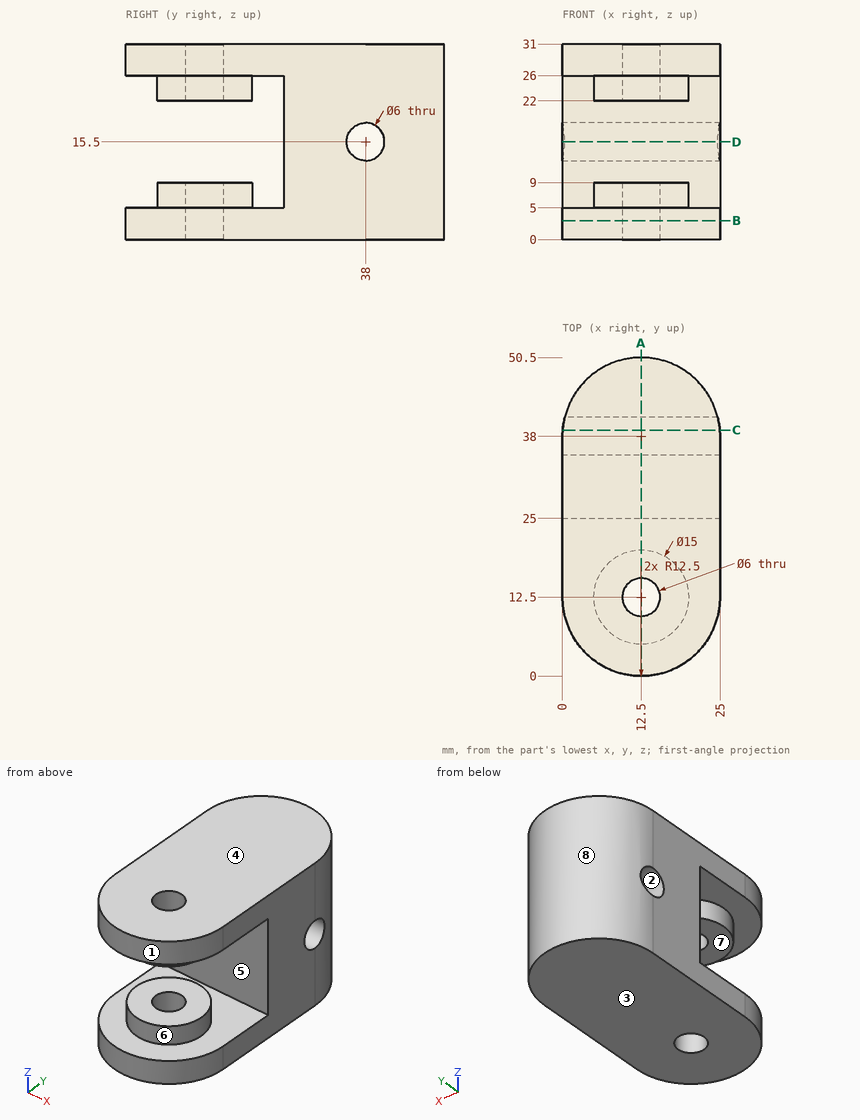
Part print with two shaded views. Sizes in mm from the minimum x, y, z corner. A direction names the side the tool comes from. Coordinates: 2 decimals unless noted, no trailing zeros. Write each loop counter-clockwise with the first axis right and the second up, starting at its lowest first coordinate (ties: lowest second). Pieces come first, ordered by that corner, then holes.
(1) Pin check, flat tips, straight feed: pin 1 Ø1 at (y, z) = (10, 26) entering from -X; pin 2 Ø5.5 at (y, z) = (38, 15.5) entering from +X; pin 3 Ø6 at (x, z) = (10, 22.5) entering from -Y. Stop position of each tip, or through.
(2) Cut at B-B on z = 3. List the corners of the cut face in (x, y), and give its area (3 significant figures).
(3) Drill centre lines: line 1 (Y direction, x = 12.5, z = 7.25); line 2 (Z direction, x = 6.25, y = 14); line 3 (Z direction, x = 20, y = 3). Where is each one in solid material? Low to high.
(4) 3-axis set-ups, long thin cutter, end or side, ignore diameter. For the marked faces 4, 5, 6, 7 and 8: which of +Z, -Z, +X, -X, +Y, -Y reach the whole face in a straight line?
(5) Mould opens along Z. For the marked faces 1, 2 and 3 say: pulls with the +Z half, pulls with the -Z half, needs draft (parallel to the pull), parting line crosses it, or undercut.
(6) Cut at D-D on z = 15.5. List the corners of the cut face in (x, y).
(7) Cut at C-C on y = 39. List the corners of the cut face in (x, z), and give its area (3 significant figures).
(8) Cut at A-A on x = 12.5. List the corners of the cut face in (y, z), and give its area (3 significant figures).
Working result:
1. pin 1: stops at x = 0.16
1. pin 2: passes through
1. pin 3: stops at y = 5
2. outline: (0, 12.5) arc R12.5 ccw to (25, 12.5) - (25, 38) arc R12.5 ccw to (0, 38) - close; hole circle Ø6 at (12.5, 12.5)
2. area: 1,100 mm2
3. line 1: y = 5 to 9.5, 15.5 to 20, 25 to 50.5
3. line 2: z = 0 to 9, 22 to 31
3. line 3: z = 0 to 5, 26 to 31
4. face 4: +Z, +X, -X, +Y, -Y
4. face 5: +X, -X
4. face 6: none
4. face 7: +X, -X, -Y
4. face 8: +Z, -Z, +Y
5. face 1: needs draft
5. face 2: undercut
5. face 3: pulls with the -Z half
6. outline: (0, 25) - (25, 25) - (25, 35) - (0, 35) - close; (0.37, 41) - (24.63, 41) arc R12.5 ccw to start
7. outline: (0.04, 0) - (24.96, 0) - (24.96, 12.67) - (0.04, 12.67) - close; (0.04, 18.33) - (24.96, 18.33) - (24.96, 31) - (0.04, 31) - close
7. area: 632 mm2
8. outline: (0, 0) - (9.5, 0) - (9.5, 9) - (5, 9) - (5, 5) - (0, 5) - close; (0, 26) - (5, 26) - (5, 22) - (9.5, 22) - (9.5, 31) - (0, 31) - close; (15.5, 0) - (50.5, 0) - (50.5, 31) - (15.5, 31) - (15.5, 22) - (20, 22) - (20, 26) - (25, 26) - (25, 5) - (20, 5) - (20, 9) - (15.5, 9) - close; hole circle Ø6 at (38, 15.5)
8. area: 1,020 mm2
